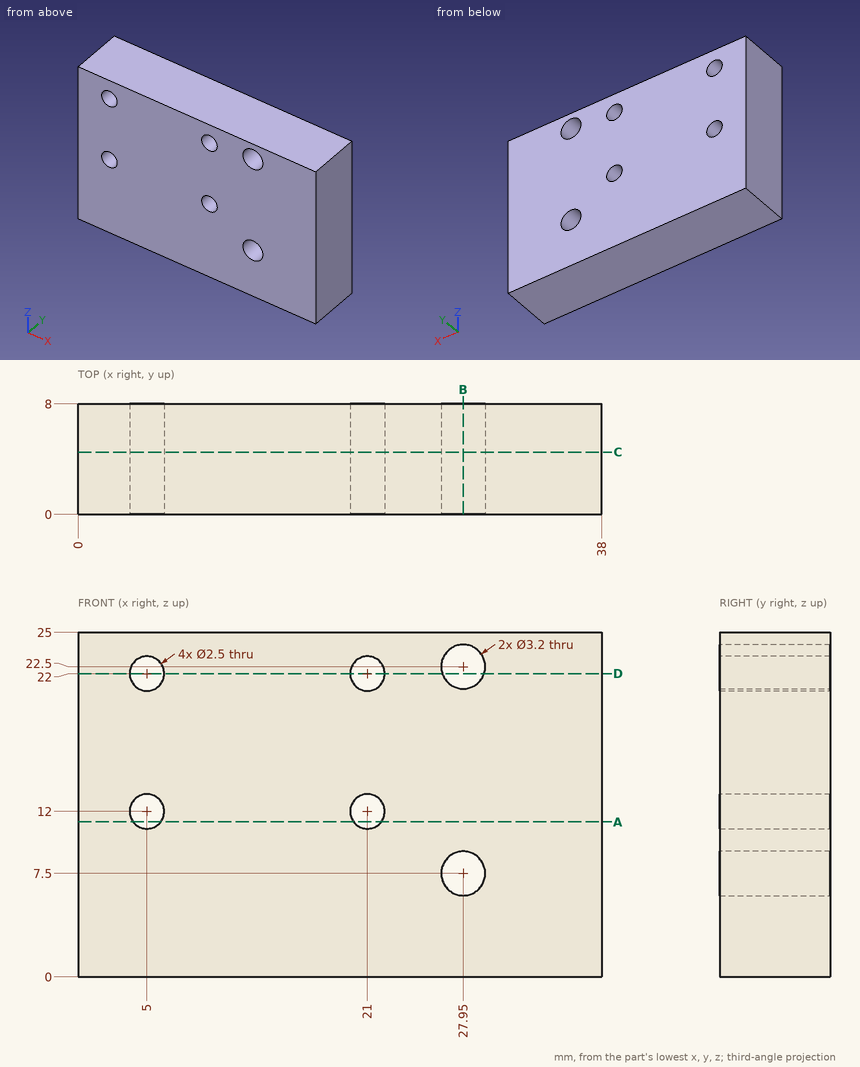
Could you check a few things on this drawing? It's one solid part, dimensions in mm from its lowest x, y, z. Coordinates: 2 decimals unless noted, no trailing zeros. Order: outer loops, then holes, each group sorted by start corner. A loop starts at its lowest first (then second) coordinate and runs counter-clockwise, first axis right, second up. Notation, with made-up numbers: (-9, -0.75) -> (18, -0.75) arc R20 cw to (18, 6.25) -> close; hole circle Ø7 at (74.25, 21.25). An arc over 180 degrees is marked (long way). Answer in a Markdown table with one row per item.
(1) I want a section at D-D on z = 22. List the corners of the cut face in (x, y) for me, then the cut area to 3 significant figures.
Answer key:
| item | result |
|---|---|
| outline | (0, 0) -> (3.75, 0) -> (3.75, 8) -> (0, 8) -> close; (6.25, 0) -> (19.75, 0) -> (19.75, 8) -> (6.25, 8) -> close; (22.25, 0) -> (26.43, 0) -> (26.43, 8) -> (22.25, 8) -> close; (29.47, 0) -> (38, 0) -> (38, 8) -> (29.47, 8) -> close |
| area | 240 mm^2 |
(2) Will this pin go through, and if not, where does the flat tip stop? pin 1 Ø1.9 at (x, z) = (27.95, 7.5) entering from -Y.
Answer key:
| item | result |
|---|---|
| pin 1 | through |
(3) Please list where these lines run through material, in increasing order: probe 1 along X at (y, z) = (4.25, 7.5); probe 2 along X at (y, z) = (3.25, 22); probe 3 along Z at (x, y) = (28.5, 7.25).
Answer key:
| item | result |
|---|---|
| probe 1 | 0 to 26.35, 29.55 to 38 |
| probe 2 | 0 to 3.75, 6.25 to 19.75, 22.25 to 26.43, 29.47 to 38 |
| probe 3 | 0 to 6, 9 to 21, 24 to 25 |
(4) I want a section at B-B on x = 27.95. List the corners of the cut face in (y, z) for me.
Answer key:
| item | result |
|---|---|
| outline | (0, 0) -> (8, 0) -> (8, 5.9) -> (0, 5.9) -> close; (0, 9.1) -> (8, 9.1) -> (8, 20.9) -> (0, 20.9) -> close; (0, 24.1) -> (8, 24.1) -> (8, 25) -> (0, 25) -> close |
(5) I want a section at C-C on y = 4.5. List the corners of the cut face in (x, z) for me.
Answer key:
| item | result |
|---|---|
| outline | (0, 0) -> (38, 0) -> (38, 25) -> (0, 25) -> close; hole circle Ø2.5 at (5, 12); hole circle Ø2.5 at (5, 22); hole circle Ø2.5 at (21, 12); hole circle Ø2.5 at (21, 22); hole circle Ø3.2 at (27.95, 7.5); hole circle Ø3.2 at (27.95, 22.5) |
(6) I want a section at A-A on z = 11.25. List the corners of the cut face in (x, y) for me.
Answer key:
| item | result |
|---|---|
| outline | (0, 0) -> (4, 0) -> (4, 8) -> (0, 8) -> close; (6, 0) -> (20, 0) -> (20, 8) -> (6, 8) -> close; (22, 0) -> (38, 0) -> (38, 8) -> (22, 8) -> close |
